Verification items for the finished model (mm, model axes). A direction names the side the tool comes from. Give positions to 0.01 mm unless a question says otherwise; leave off trailing zeros. Write each loop counter-clockwise with the first axis right and the second up, starting at its lowest first coordinate (ties: lowest second). Pieces come first, ordered by that corner, then holes. Notation, with made-up numbers: (26.5, -11) -> (71.5, -11) arc R28 cw to (71.5, 23) -> close; hole circle Ø3 at (-34, 59.5). An arc over 180 degrees is marked (long way). Write item = value, one per line.
from build123d import *

# Parameters (mm, degrees)
SKETCH1_R           = 1.6891
SKETCH1_R_2         = 1.905
BOSS_EXTRUDE1_DEPTH = 4


with BuildPart() as part:
    # Sketch1 → Boss-Extrude1 (new body)
    with BuildSketch(Plane(origin=(0, 0, 0), x_dir=(1, 0, 0), z_dir=(0, 1, 0))):
        Polygon((28.575, 215.9), (28.575, 0), (282.575, 0), (282.575, 254), (28.575, 254), align=None)
        with Locations(Location((47.625, 25.4, 0), (0, 0, 270))):
            Circle(SKETCH1_R, mode=Mode.SUBTRACT)
        with BuildLine():
            Line((184.540258822, 41.0845), (155.163048801, 41.0845))
            Line((155.163048801, 41.0845), (126.602331606, 41.0845))
            ThreePointArc((126.602331606, 41.0845), (126.776599265, 40.735252505), (126.836576836, 40.349576836))
            ThreePointArc((126.836576836, 40.349576836), (124.678175908, 39.442028606), (125.5395, 41.61928816))
            Line((125.5395, 41.61928816), (125.5395, 97.69971184))
            ThreePointArc((125.5395, 97.69971184), (124.678175908, 99.876971394), (126.836576836, 98.969423164))
            ThreePointArc((126.836576836, 98.969423164), (126.712192056, 98.421275585), (126.363402398, 97.9805))
            Line((126.363402398, 97.9805), (184.786597602, 97.9805))
            ThreePointArc((184.786597602, 97.9805), (185.035275585, 100.115038384), (186.853423164, 98.969423164))
            ThreePointArc((186.853423164, 98.969423164), (186.490971394, 98.081022236), (185.6105, 97.69971184))
            Line((185.6105, 97.69971184), (185.6105, 41.589727831))
            ThreePointArc((185.6105, 41.589727831), (186.472493583, 41.199152325), (186.825084987, 40.320937393))
            ThreePointArc((186.825084987, 40.320937393), (185.152548795, 39.116418977), (184.540258822, 41.0845))
        make_face(mode=Mode.SUBTRACT)
        with Locations(Location((263.525, 25.4, 0), (0, 0, 270))):
            Circle(SKETCH1_R, mode=Mode.SUBTRACT)
        with BuildLine():
            Line((82.477295998, 189.534156397), (84.382295998, 189.534156397))
            Line((84.382295998, 189.534156397), (86.287295998, 189.534156397))
            Line((86.287295998, 189.534156397), (86.287295998, 187.197356397))
            ThreePointArc((86.287295998, 187.197356397), (93.970795998, 177.8), (86.287295998, 168.402643603))
            Line((86.287295998, 168.402643603), (86.287295998, 166.1795))
            Line((86.287295998, 166.1795), (84.382295998, 166.1795))
            Line((84.382295998, 166.1795), (82.477295998, 166.1795))
            Line((82.477295998, 166.1795), (82.477295998, 168.402643603))
            ThreePointArc((82.477295998, 168.402643603), (77.30886259, 171.326525503), (74.853325959, 176.7332))
            Line((74.853325959, 176.7332), (73.701595998, 176.7332))
            Line((73.701595998, 176.7332), (73.701595998, 177.8))
            Line((73.701595998, 177.8), (73.701595998, 178.8668))
            Line((73.701595998, 178.8668), (74.853325959, 178.8668))
            ThreePointArc((74.853325959, 178.8668), (77.30886259, 184.273474497), (82.477295998, 187.197356397))
            Line((82.477295998, 187.197356397), (82.477295998, 189.534156397))
        make_face(mode=Mode.SUBTRACT)
        with Locations(Location((108.760866591, 138.366268292, 0), (0, 0, 270))):
            Circle(SKETCH1_R_2, mode=Mode.SUBTRACT)
        Polygon((106.8705, 185.6994), (155.575, 185.6994), (204.1525, 185.6994), (204.1525, 145.7452), (106.8705, 145.7452), align=None, mode=Mode.SUBTRACT)
        with Locations(Location((47.625, 224.852960253, 0), (0, 0, 270))):
            Circle(SKETCH1_R, mode=Mode.SUBTRACT)
        with Locations(Location((108.760866591, 193.767535109, 0), (0, 0, 270))):
            Circle(SKETCH1_R_2, mode=Mode.SUBTRACT)
        with Locations(Location((202.643133409, 138.366268292, 0), (0, 0, 270))):
            Circle(SKETCH1_R_2, mode=Mode.SUBTRACT)
        with Locations(Location((202.643133409, 193.767535109, 0), (0, 0, 270))):
            Circle(SKETCH1_R_2, mode=Mode.SUBTRACT)
        with Locations(Location((263.525, 224.852960253, 0), (0, 0, 270))):
            Circle(SKETCH1_R, mode=Mode.SUBTRACT)
    extrude(amount=BOSS_EXTRUDE1_DEPTH)


solid = part.part
Item 1: Sectioned sample at B-B on z = -152. Record the cut outline in (x, y) (1 decimal).
Response values:
outline = (28.6, 0) -> (106.9, 0) -> (106.9, 4) -> (28.6, 4) -> close; (204.2, 0) -> (282.6, 0) -> (282.6, 4) -> (204.2, 4) -> close
Item 2: Sectioned sample at A-A on x = 115. Record the cut outline in (y, z), then the cut area to 3 significant figures.
Response values:
outline = (0, -254) -> (4, -254) -> (4, -185.7) -> (0, -185.7) -> close; (0, -145.75) -> (4, -145.75) -> (4, 0) -> (0, 0) -> close
area = 856 mm^2
Item 3: Sectioned sample at C-C on y = 2.35. Give the number of separate pieces and of enclosed holes in the cut face, then the cut area to 3 significant figures.
Response values:
separate_pieces = 1
enclosed_holes = 11
area = 56,800 mm^2
Item 4: Go/stop test with flat-tipped pins: P1, Ø4.5, axis at x = 202.64, z = -138.37, coming from the +Y side; P2, Ø2.5, axis at x = 47.62, z = -224.85, coming from the -Y side. Record where each tip stops, or that it passes through.
Response values:
P1 = 4
P2 = through
Item 5: Mould release check, pull along X, two halves, no side actions. Record for faces 1 (the cylindrical face through (77.37, 1.97, -171.26)), 2 (the flat face through (154, 0, -129)): +X half, -X half, draft (parallel to the pull), parting line (faces both ways), or undercut.
Response values:
face_1 = undercut
face_2 = draft
Item 6: Set-up check for faces 3 (the flat face through (154, 4, -129)), 4 (the cylindrical face through (77.25, 1.97, -184.21)): record each of +Z, -Z, +X, -X, +Y, -Y from which the full face is reachable in a straight line by a thin tool's end or side.
Response values:
face_3 = +Z, -Z, +X, -X, +Y
face_4 = +Y, -Y
Item 7: Material ranges on line 1 (X direction, y = 2.95, z = -25.4) (3 decimals); line 2 (Z direction, x = 122, y = 0.6); line 3 (X direction, y = 2.6, z = -97) (1 decimal), recorded low to high.
Response values:
line_1 = 28.575 to 45.936, 49.314 to 261.836, 265.214 to 282.575
line_2 = -254 to -185.7, -145.75 to 0
line_3 = 28.6 to 125.5, 185.6 to 282.6
